Could you check a few things on this model? Use its own coordinates, in mm. Face numbers are marked on the shaded views. Round coordinates to 2 decimals unless told otherwise and drop trailing zeros. Loops run counter-clockwise (first coordinate to the right, second up) from the corner with the lowest first, then second, coordinate; pieces in that order, holes last. Notation, with made-up numbers: (27.25, 87) -> (42.25, 87) arc R15 ccw to (42.25, 115) -> close; hole circle Ø6 at (88, -4). An arc over 180 degrees is marked (long way). One line per item, written item: value.
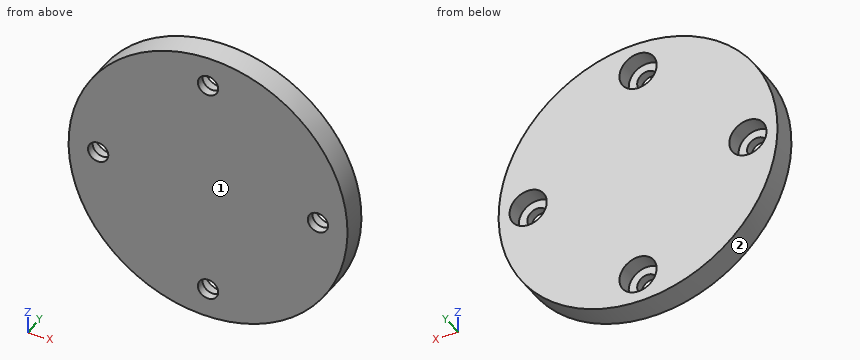
```python
from build123d import *

# Parameters (mm, degrees)
SKETCH1_R                      = 16.5
BOSS_EXTRUDE1_DEPTH            = 3
CBORE_FOR_M2_SHCS1_D           = 2.4
CBORE_FOR_M2_SHCS1_CBORE_D     = 4.4
CBORE_FOR_M2_SHCS1_CBORE_DEPTH = 2
CIRPATTERN1_COUNT              = 4


with BuildPart() as part:
    # Sketch1 → Boss-Extrude1 (new body)
    with BuildSketch(Plane(origin=(0, 0, 0), x_dir=(1, 0, 0), z_dir=(0, 1, 0))):
        with Locations(Location((0, 0, 0), (0, 0, 270))):
            Circle(SKETCH1_R)
    extrude(amount=BOSS_EXTRUDE1_DEPTH)

    # CBORE for M2 SHCS1 (through all)
    with Locations(Plane(origin=(0, 3, 0), x_dir=(1, 0, 0), z_dir=(0, 1, 0))):
        with Locations((-13, 0)):
            cbore_for_m2_shcs1 = CounterBoreHole(CBORE_FOR_M2_SHCS1_D / 2, CBORE_FOR_M2_SHCS1_CBORE_D / 2, CBORE_FOR_M2_SHCS1_CBORE_DEPTH)

    # CirPattern1: CBORE for M2 SHCS1 ×4 about axis
    cirpattern1_axis = Axis((0, 0, 0), (0, 1, 0))
    for i in range(1, CIRPATTERN1_COUNT):
        add(cbore_for_m2_shcs1.rotate(cirpattern1_axis, i * 360 / CIRPATTERN1_COUNT), mode=Mode.SUBTRACT)


solid = part.part
```
Item 1: If we section it at D-D on x = -0.5: List the corners of the cut face in (y, z) for me, plus the area to 3 significant figures.
Output:
outline: (0, -16.49) -> (3, -16.49) -> (3, -15.14) -> (1, -15.14) -> (1, -14.09) -> (0, -14.09) -> close; (0, -11.91) -> (1, -11.91) -> (1, -10.86) -> (3, -10.86) -> (3, 10.86) -> (1, 10.86) -> (1, 11.91) -> (0, 11.91) -> close; (0, 14.09) -> (1, 14.09) -> (1, 15.14) -> (3, 15.14) -> (3, 16.49) -> (0, 16.49) -> close
area: 77.5 mm²
Item 2: If we section it at B-B on x = -12.5: List the corners of the cut face in (y, z) for me, plus the area to 3 significant figures.
Output:
outline: (0, -10.77) -> (3, -10.77) -> (3, -2.14) -> (1, -2.14) -> (1, -1.09) -> (0, -1.09) -> close; (0, 1.09) -> (1, 1.09) -> (1, 2.14) -> (3, 2.14) -> (3, 10.77) -> (0, 10.77) -> close
area: 53.9 mm²
Item 3: If we section it at A-A on z = 0: List the corners of the cut face in (x, y) for me.
Output:
outline: (-16.5, 0) -> (-14.2, 0) -> (-14.2, 1) -> (-15.2, 1) -> (-15.2, 3) -> (-16.5, 3) -> close; (-11.8, 0) -> (11.8, 0) -> (11.8, 1) -> (10.8, 1) -> (10.8, 3) -> (-10.8, 3) -> (-10.8, 1) -> (-11.8, 1) -> close; (14.2, 0) -> (16.5, 0) -> (16.5, 3) -> (15.2, 3) -> (15.2, 1) -> (14.2, 1) -> close
Item 4: I need wall thicknesses on line 1 (Z direction, x = 13, y = 2.6); line 2 (Z direction, x = -12, y = 2); line 3 (X direction, y = 1.2, z = -12.5). Which ranges of each line are inside material? Lowest first, please. Write a range as from..to.
Output:
line 1: z = -10.16..-2.2, 2.2..10.16
line 2: z = -11.32..-1.96, 1.96..11.32
line 3: x = -10.77..-2.14, 2.14..10.77
Item 5: If we section it at C-C on y = 1.8: List the corners of the cut face in (x, z) for me, plus the area to 3 significant figures.
Output:
outline: circle Ø33 at (0, 0); hole circle Ø4.4 at (-13, 0); hole circle Ø4.4 at (0, -13); hole circle Ø4.4 at (0, 13); hole circle Ø4.4 at (13, 0)
area: 794 mm²
Item 6: Will these pins go through, and if not, where does the flat tip stop? pin 1 Ø1.5 at (x, y) = (12, 1) entering from -Z; pin 2 Ø1.3 at (x, z) = (1, 14) entering from +Y; pin 3 Ø1.5 at (x, y) = (1, 1.5) entering from -Z.
Output:
pin 1: stops at z = -12.07
pin 2: stops at y = 1
pin 3: stops at z = -16.5
Item 7: If we mould it in two halves opening along Z, with no side actions, what happens to the marked faces 1 and 2? For each: released by +Z, released by -Z, zero draft, split by the parting line, or undercut.
Output:
face 1: zero draft
face 2: split by the parting line
